Geometry check sheet. Reference: the model listing, model coordinates, mm. Face numbers are marked on the shaded views. A direction names the side the tool comes from. Round coordinates to 2 decimals unless told otherwise and drop trailing zeros. Order: outer loops, then holes, each group sorted by start corner. A loop starts at its lowest first (then second) coordinate and runs counter-clockwise, first axis right, second up. Notation, with made-up numbers: (-23, 88.5) - (29, 88.5) arc R12 ccw to (29, 109.5) - close; hole circle Ø10 at (-21, 19.5). An arc over 180 degrees is marked (long way). Use a Markdown table: item, result. Add a question column.
(1) Section check A-A on y = 69.5. Record the boundary of the cut face in (x, z), then the cut area to 3 significant figures.
(2) Section check B-B on z = 4. Give the number of separate pieces and of enclosed holes in the cut face, then the cut area to 3 significant figures.
(3) Gauge pin test, flat ends, axial feed: P1, Ø1, axis at x = 8.5, z = 2, coming from the +Y side; P2, Ø1.5, axis at y = 35.5, z = 3.5, coming from the +X side; P3, Ø1.8, axis at y = 107, z = 4, coming from the +X side. Record the tip position at first contact, or that the pin passes through.
(4) Mould release check, pull along Y, two halves, no side actions. Record for the marked faces 3, 4 and 5: released by +Y, released by -Y, zero draft, split by the parting line, or undercut.
(5) Access from +Z, -Z, +X, -X, +Y, -Y to the whole of each face (thin tool, end or side, straight path). Record for the marked faces 1 and 2.
(6) Thickness scan on line 1 along X through (y, z) = (47.5, 1.5); line 2 along Y through (x, z) = (-16, 2.5); line 3 along X through (y, z) = (-7.5, 3.75). Record the ranges inside material, lowest first. Write a range as [from, to].
```python
from build123d import *

# Parameters (mm, degrees)
SKETCH1_R               = 7.95
SKETCH1_R_2             = 3
MAIN_BODY_LINK_B1_DEPTH = 6
CUT_EXTRUDE2_REACH      = 169.025
CUT_EXTRUDE3_REACH      = 169.025
SKETCH5_R               = 1.5
PULLEYIDLERUP_DEPTH     = 6
CUT_EXTRUDE5_DEPTH      = 6
FILLET4_R               = 1
FILLET5_R               = 100
SKETCH8_R               = 15.25
CUT_EXTRUDE6_DEPTH      = 168.02546447


with BuildPart() as part:
    # Sketch1 → Main Body Link B1 (new body)
    with BuildSketch(Plane.XY):
        with BuildLine():
            Line((20.2, 41.674052381), (20.2, 83.474052381))
            Line((20.2, 83.474052381), (20.2, 90.874052381))
            Line((20.2, 90.874052381), (17.986683974, 148.383116621))
            ThreePointArc((17.986683974, 148.383116621), (0, 165.690874165), (-17.986683974, 148.383116621))
            Line((-17.986683974, 148.383116621), (-20.2, 90.874052381))
            Line((-20.2, 90.874052381), (-20.2, 83.474052381))
            Line((-20.2, 83.474052381), (-20.2, 41.674052381))
            Line((-20.2, 41.674052381), (-20.2, 34.274052381))
            Line((-20.2, 34.274052381), (-17.964224051, -1.134307826))
            ThreePointArc((-17.964224051, -1.134307826), (0, -18), (17.964224051, -1.134307826))
            Line((17.964224051, -1.134307826), (20.2, 34.274052381))
            Line((20.2, 34.274052381), (20.2, 41.674052381))
        make_face()
        Circle(SKETCH1_R, mode=Mode.SUBTRACT)
        with Locations((15, 88.174052381)):
            Circle(SKETCH1_R_2, mode=Mode.SUBTRACT)
        with Locations((-15, 37.024052381)):
            Circle(SKETCH1_R_2, mode=Mode.SUBTRACT)
        with Locations((0, 147.690874165)):
            Circle(SKETCH1_R, mode=Mode.SUBTRACT)
    extrude(amount=MAIN_BODY_LINK_B1_DEPTH)

    # Sketch4 → Cut-Extrude2 (cut, up to next)
    with BuildSketch(Plane.XY.offset(6), mode=Mode.PRIVATE) as cut_extrude2_sk1:
        with BuildLine():
            Line((-12, 134.2744663), (-12, 123.584968066))
            Line((-12, 123.584968066), (-2.929911079, 129.930929878))
            ThreePointArc((-2.929911079, 129.930929878), (-7.774454217, 131.456408925), (-12, 134.2744663))
        make_face()
    cut_extrude2_tool1 = extrude(cut_extrude2_sk1.sketch, amount=-CUT_EXTRUDE2_REACH, mode=Mode.PRIVATE) & part.part
    # Sketch4 → Cut-Extrude2 (cut, up to next)
    with BuildSketch(Plane.XY.offset(6), mode=Mode.PRIVATE) as cut_extrude2_sk2:
        Polygon((-12, 100.690874165), (3.278172542, 100.690874165), (-12, 111.380372399), align=None)
    cut_extrude2_tool2 = extrude(cut_extrude2_sk2.sketch, amount=-CUT_EXTRUDE2_REACH, mode=Mode.PRIVATE) & part.part
    # Sketch4 → Cut-Extrude2 (cut, up to next)
    with BuildSketch(Plane.XY.offset(6), mode=Mode.PRIVATE) as cut_extrude2_sk3:
        Polygon((12, 128.172168466), (12, 106.793171999), (-3.278172542, 117.482670232), align=None)
    cut_extrude2_tool3 = extrude(cut_extrude2_sk3.sketch, amount=-CUT_EXTRUDE2_REACH, mode=Mode.PRIVATE) & part.part
    # Sketch4 → Cut-Extrude2 (cut, up to next)
    with BuildSketch(Plane.XY.offset(6), mode=Mode.PRIVATE) as cut_extrude2_sk4:
        Polygon((-4.386441158, 88.090874165), (12, 88.090874165), (12, 73.82101499), align=None)
    cut_extrude2_tool4 = extrude(cut_extrude2_sk4.sketch, amount=-CUT_EXTRUDE2_REACH, mode=Mode.PRIVATE) & part.part
    # Sketch4 → Cut-Extrude2 (cut, up to next)
    with BuildSketch(Plane.XY.offset(6), mode=Mode.PRIVATE) as cut_extrude2_sk5:
        Polygon((-12, 81.46073334), (-12, 52.92101499), (4.386441158, 67.190874165), align=None)
    cut_extrude2_tool5 = extrude(cut_extrude2_sk5.sketch, amount=-CUT_EXTRUDE2_REACH, mode=Mode.PRIVATE) & part.part
    # Sketch4 → Cut-Extrude2 (cut, up to next)
    with BuildSketch(Plane.XY.offset(6), mode=Mode.PRIVATE) as cut_extrude2_sk6:
        Polygon((-4.386441158, 46.290874165), (12, 46.290874165), (12, 60.56073334), align=None)
    cut_extrude2_tool6 = extrude(cut_extrude2_sk6.sketch, amount=-CUT_EXTRUDE2_REACH, mode=Mode.PRIVATE) & part.part
    add(cut_extrude2_tool1.solids().sort_by_distance((-9.12997, 128.978342, 6))[0], mode=Mode.SUBTRACT)
    add(cut_extrude2_tool2.solids().sort_by_distance((-6.907276, 104.25404, 6))[0], mode=Mode.SUBTRACT)
    add(cut_extrude2_tool3.solids().sort_by_distance((6.907276, 117.48267, 6))[0], mode=Mode.SUBTRACT)
    add(cut_extrude2_tool4.solids().sort_by_distance((6.537853, 83.334254, 6))[0], mode=Mode.SUBTRACT)
    add(cut_extrude2_tool5.solids().sort_by_distance((-6.537853, 67.190874, 6))[0], mode=Mode.SUBTRACT)
    add(cut_extrude2_tool6.solids().sort_by_distance((6.537853, 51.047494, 6))[0], mode=Mode.SUBTRACT)

    # Sketch5 → Cut-Extrude3 (cut, up to next)
    with BuildSketch(Plane.XY.offset(6), mode=Mode.PRIVATE) as cut_extrude3_sk1:
        with Locations((11.5, 147.690874165)):
            Circle(SKETCH5_R)
    cut_extrude3_tool1 = extrude(cut_extrude3_sk1.sketch, amount=-CUT_EXTRUDE3_REACH, mode=Mode.PRIVATE) & part.part
    # Sketch5 → Cut-Extrude3 (cut, up to next)
    with BuildSketch(Plane.XY.offset(6), mode=Mode.PRIVATE) as cut_extrude3_sk2:
        with Locations((-11.5, 147.690874165)):
            Circle(SKETCH5_R)
    cut_extrude3_tool2 = extrude(cut_extrude3_sk2.sketch, amount=-CUT_EXTRUDE3_REACH, mode=Mode.PRIVATE) & part.part
    # Sketch5 → Cut-Extrude3 (cut, up to next)
    with BuildSketch(Plane.XY.offset(6), mode=Mode.PRIVATE) as cut_extrude3_sk3:
        with Locations((-11.5, 0)):
            Circle(SKETCH5_R)
    cut_extrude3_tool3 = extrude(cut_extrude3_sk3.sketch, amount=-CUT_EXTRUDE3_REACH, mode=Mode.PRIVATE) & part.part
    # Sketch5 → Cut-Extrude3 (cut, up to next)
    with BuildSketch(Plane.XY.offset(6), mode=Mode.PRIVATE) as cut_extrude3_sk4:
        with Locations((11.5, 0)):
            Circle(SKETCH5_R)
    cut_extrude3_tool4 = extrude(cut_extrude3_sk4.sketch, amount=-CUT_EXTRUDE3_REACH, mode=Mode.PRIVATE) & part.part
    add(cut_extrude3_tool1.solids().sort_by_distance((11.5, 147.690874, 6))[0], mode=Mode.SUBTRACT)
    add(cut_extrude3_tool2.solids().sort_by_distance((-11.5, 147.690874, 6))[0], mode=Mode.SUBTRACT)
    add(cut_extrude3_tool3.solids().sort_by_distance((-11.5, 0, 6))[0], mode=Mode.SUBTRACT)
    add(cut_extrude3_tool4.solids().sort_by_distance((11.5, 0, 6))[0], mode=Mode.SUBTRACT)

    # Sketch6 → PulleyIdlerUp (cut)
    with BuildSketch(Plane.XY.offset(6)):
        with BuildLine():
            Line((-5.672455467, 109.394173307), (6.61799676, 100.795058))
            ThreePointArc((6.61799676, 100.795058), (10.795910267, 101.533325384), (10.057642883, 105.71123889))
            Line((10.057642883, 105.71123889), (-2.232809344, 114.310354197))
            ThreePointArc((-2.232809344, 114.310354197), (-6.410722851, 113.572086814), (-5.672455467, 109.394173307))
        make_face()
    extrude(amount=-PULLEYIDLERUP_DEPTH, mode=Mode.SUBTRACT)

    # Sketch7 → Cut-Extrude5 (cut)
    with BuildSketch(Plane.XY.offset(6)):
        with BuildLine():
            Line((-11.550553841, 24.425461103), (0.736726824, 15.821814558))
            ThreePointArc((0.736726824, 15.821814558), (4.914912266, 16.558541382), (4.178185442, 20.736726824))
            Line((4.178185442, 20.736726824), (-8.109095222, 29.340373369))
            ThreePointArc((-8.109095222, 29.340373369), (-12.287280664, 28.603646545), (-11.550553841, 24.425461103))
        make_face()
    extrude(amount=-CUT_EXTRUDE5_DEPTH, mode=Mode.SUBTRACT)

    # Fillet4
    fillet4_edges = [part.edges().sort_by_distance(p)[0] for p in [
        (-12, 81.46073334, 3),
        (4.386441158, 67.190874165, 3),
        (-12, 52.92101499, 3),
        (-12, 134.2744663, 3),
        (-2.929911079, 129.930929878, 3),
        (-12, 123.584968066, 3),
        (-12, 100.690874165, 3),
        (-12, 111.380372399, 3),
        (3.278172542, 100.690874165, 3),
        (12, 106.793171999, 3),
        (-3.278172542, 117.482670232, 3),
        (12, 128.172168466, 3),
        (12, 60.56073334, 3),
        (12, 46.290874165, 3),
        (-4.386441158, 46.290874165, 3),
        (12, 88.090874165, 3),
        (12, 73.82101499, 3),
        (-4.386441158, 88.090874165, 3),
    ]]
    fillet(fillet4_edges, radius=FILLET4_R)

    # Fillet5
    # the kernel refuses this fillet: 100 mm, written as the material it takes off along each edge
    with BuildSketch(Plane(origin=(-20.2, 34.274052381, -7.884973578), x_dir=(0, 1, 0), z_dir=(0, 0, 1))) as fillet5_piece_1:
        with BuildLine():
            CenterArc((FILLET5_R * 0.0315398943126, -FILLET5_R), FILLET5_R, 90, 3.613007947)
            Line((-FILLET5_R * 0.0314772071099, -FILLET5_R * 0.00198755271875), (0, 0))
            Line((0, 0), (FILLET5_R * 0.0315398943126, 0))
        make_face()
    extrude(amount=21.769947156, mode=Mode.SUBTRACT)
    with BuildSketch(Plane(origin=(-20.2, 90.874052381, -4.809018086), x_dir=(0.03845791424359976, 0.9992602207793684, 0), z_dir=(0, 0, 1))) as fillet5_piece_2:
        with BuildLine():
            CenterArc((FILLET5_R * 0.0192360723451, -FILLET5_R), FILLET5_R, 90, 2.204019698)
            Line((-FILLET5_R * 0.0192218418985, -FILLET5_R * 0.000739779220632), (0, 0))
            Line((0, 0), (FILLET5_R * 0.0192360723451, 0))
        make_face()
    extrude(amount=15.618036173, mode=Mode.SUBTRACT)
    with BuildSketch(Plane(origin=(20.2, 90.874052381, -4.809018086), x_dir=(-0.03845791424359111, 0.9992602207793686, 0), z_dir=(0, 0, 1))) as fillet5_piece_3:
        with BuildLine():
            CenterArc((FILLET5_R * 0.0192360723451, FILLET5_R), FILLET5_R, 267.795980302, 2.204019698)
            Line((-FILLET5_R * 0.0192218418985, FILLET5_R * 0.000739779220631), (0, 0))
            Line((0, 0), (FILLET5_R * 0.0192360723451, 0))
        make_face()
    extrude(amount=15.618036173, mode=Mode.SUBTRACT)
    with BuildSketch(Plane(origin=(20.2, 34.274052381, -7.884973578), x_dir=(0, 1, 0), z_dir=(0, 0, 1))) as fillet5_piece_4:
        with BuildLine():
            CenterArc((FILLET5_R * 0.0315398943126, FILLET5_R), FILLET5_R, 266.386992053, 3.613007947)
            Line((-FILLET5_R * 0.0314772071099, FILLET5_R * 0.00198755271875), (0, 0))
            Line((0, 0), (FILLET5_R * 0.0315398943126, 0))
        make_face()
    extrude(amount=21.769947156, mode=Mode.SUBTRACT)

    # Sketch8 → Cut-Extrude6 (cut, through all)
    with BuildSketch(Plane.XY.offset(6)):
        Circle(SKETCH8_R)
        with Locations((0, 147.690874165)):
            Circle(SKETCH8_R)
    extrude(amount=-CUT_EXTRUDE6_DEPTH, mode=Mode.SUBTRACT)


solid = part.part
```
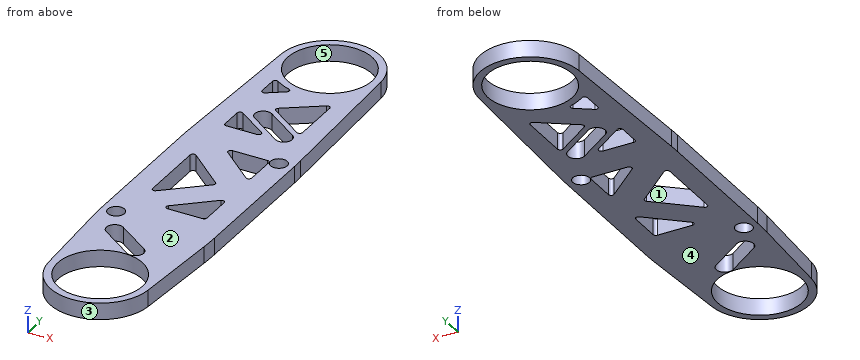
Check sheet entries:
| question | item | result |
|---|---|---|
| 1 | outline | (-20.2, 0) - (-12, 0) - (-12, 6) - (-20.2, 6) - close; (1.73, 0) - (20.2, 0) - (20.2, 6) - (1.73, 6) - close |
| 1 | area | 160 mm2 |
| 2 | separate pieces | 1 |
| 2 | enclosed holes | 12 |
| 2 | area | 4,290 mm2 |
| 3 | P1 | stops at y = 163.82 |
| 3 | P2 | stops at x = 20.19 |
| 3 | P3 | stops at x = 19.61 |
| 4 | face 3 | released by -Y |
| 4 | face 4 | zero draft |
| 4 | face 5 | undercut |
| 5 | face 1 | +Z, -Z |
| 5 | face 2 | +Z, +X, -X, +Y, -Y |
| 6 | line 1 | x = [-20.2, -2.69], [12, 20.2] |
| 6 | line 2 | y = [-8.25, 34.2], [39.85, 155.94] |
| 6 | line 3 | x = [-16.36, -13.28], [13.28, 16.36] |
